Could you check a few things on this model? Use its own coordinates, in mm. Face numbers are marked on the shaded views. A direction names the side the tool comes from. Round coordinates to 2 decimals unless told otherwise and drop trailing zeros. Loops run counter-clockwise (first coordinate to the right, second up) from the corner with the lowest first, then second, coordinate; pieces in that order, holes last.
from build123d import *

# Parameters (mm, degrees)
BOSS_EXTRUDE1_DEPTH = 20
SKETCH5_W           = 39
SKETCH5_H           = 32
CUT_EXTRUDE1_DEPTH  = 98.75607398
SKETCH6_W           = 59
SKETCH6_H           = 54.995658629
CUT_EXTRUDE2_DEPTH  = 15
SKETCH7_W           = 115
SKETCH7_H           = 80
CUT_EXTRUDE3_DEPTH  = 15
SKETCH8_OUTSIDE_W   = 145.484
SKETCH8_OUTSIDE_H   = 60.484
CUT_EXTRUDE4_DEPTH  = 170.576678821


with BuildPart() as part:
    # Sketch1 → Boss-Extrude1 (new body)
    with BuildSketch(Plane(origin=(0, 0, 0), x_dir=(1, 0, 0), z_dir=(0, 1, 0))):
        with BuildLine():
            Line((40, -52.5), (-40, -52.5))
            ThreePointArc((-40, -52.5), (-68.284271247, -40.784271247), (-80, -12.5))
            Line((-80, -12.5), (-80, 12.5))
            ThreePointArc((-80, 12.5), (-68.284271247, 40.784271247), (-40, 52.5))
            Line((-40, 52.5), (40, 52.5))
            ThreePointArc((40, 52.5), (68.284271247, 40.784271247), (80, 12.5))
            Line((80, 12.5), (80, -12.5))
            ThreePointArc((80, -12.5), (68.284271247, -40.784271247), (40, -52.5))
        make_face()
    extrude(amount=BOSS_EXTRUDE1_DEPTH)

    # Sketch5 → Cut-Extrude1 (cut, through all)
    with BuildSketch(Plane(origin=(0, 20, 0), x_dir=(1, 0, 0), z_dir=(0, 1, 0))):
        with Locations((-0.079334532, -24.5)):
            Rectangle(SKETCH5_W, SKETCH5_H)
    extrude(amount=-CUT_EXTRUDE1_DEPTH, mode=Mode.SUBTRACT)

    # Sketch6 → Cut-Extrude2 (cut)
    with BuildSketch(Plane.XZ):
        with Locations((-0.079334532, 15.997829315)):
            Rectangle(SKETCH6_W, SKETCH6_H)
    extrude(amount=-CUT_EXTRUDE2_DEPTH, mode=Mode.SUBTRACT)

    # Sketch7 → Cut-Extrude3 (cut)
    with BuildSketch(Plane.XZ):
        Rectangle(SKETCH7_W, SKETCH7_H)
    extrude(amount=-CUT_EXTRUDE3_DEPTH, mode=Mode.SUBTRACT)

    # Sketch8 outside → Cut-Extrude4 (cut, through all)
    with BuildSketch(Plane(origin=(80, 0, 0), x_dir=(0, 0, -1), z_dir=(1, 0, 0))):
        with Locations((0, 10)):
            Rectangle(SKETCH8_OUTSIDE_W, SKETCH8_OUTSIDE_H)
        Polygon((0, 20), (52.5, 7.5), (52.5, 0), (-27.5, 0), (-52.5, 0), (-52.5, 20), (-27.5, 20), align=None, mode=Mode.SUBTRACT)
    extrude(amount=-CUT_EXTRUDE4_DEPTH, mode=Mode.SUBTRACT)


solid = part.part
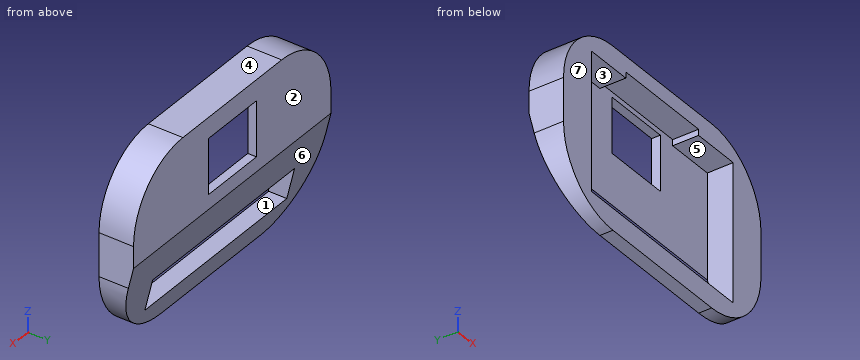
Item 1: Will these pins go through, and if not, where does the flat tip stop? pin 1 (4.5 mm diameter, centred on x = -44, y = 6.5, fed in from -Z); pin 2 (4 mm diameter, centred on y = 16.5, z = 26, fed in from +X); pin 3 (12 mm diameter, centred on y = 16, z = 38.5, fed in from -X).
Results list:
pin 1: stops at z = -52.46
pin 2: stops at x = 78.31
pin 3: stops at x = -74.64
Item 2: If we section it at B-B, the plane x = -37.5: Please give me the cut outline in (y, z).
Results list:
outline: (0, -52.5) - (7.5, -52.5) - (10.48, -40) - (0, -40) - close; (0, 40) - (15, 40) - (15, -21) - (20, 0) - (20, 52.5) - (0, 52.5) - close
Item 3: For the marked faces 1, 2 and 3, which set-ups out of +Z, -Z, +X, -X, +Y, -Y let a thin tool reach every point of the face, with its end or its side?
Results list:
face 1: +Y, -Y
face 2: +Z, -Z, +X, -X, +Y
face 3: -Y
Item 4: If we section it at A-A, the plane x = 4: Please give me the cut outline in (y, z), then the cut area to 3 significant figures.
Results list:
outline: (0, -52.5) - (7.5, -52.5) - (10.48, -40) - (0, -40) - close; (0, 43.5) - (15, 43.5) - (15, 40.5) - (20, 40.5) - (20, 52.5) - (0, 52.5) - close; (15, -21) - (20, 0) - (20, 8.5) - (15, 8.5) - close
area: 402 mm2
Item 5: If we section it at D-D, the plane z = -35: Please give me the cut outline in (x, y).
Results list:
outline: (-73.07, 0) - (-57.5, 0) - (-57.5, 11.67) - (-73.07, 11.67) - close; (57.5, 0) - (73.07, 0) - (73.07, 11.67) - (57.5, 11.67) - close
Item 6: If we section it at C-C, the plane y = 2.5: Please give me the cut outline in (x, z), then the cut area to 3 significant figures.
Results list:
outline: (-80, -12.5) arc R40 ccw to (-40, -52.5) - (40, -52.5) arc R40 ccw to (80, -12.5) - (80, 12.5) arc R40 ccw to (40, 52.5) - (-40, 52.5) arc R40 ccw to (-80, 12.5) - close; hole (-57.5, -40) - (57.5, -40) - (57.5, 40) - (29.42, 40) - (29.42, 43.5) - (-29.58, 43.5) - (-29.58, 40) - (-57.5, 40) - close
area: 6,020 mm2
Item 7: If I drill on line 1 along X through (y, z) = (3.75, 6.5); line 2 along Z through (x, y) = (-25, 2.5); line 3 along X through (y, z) = (10.5, -26), over which ranges is the centre line in solid material (lowest first)?
Results list:
line 1: x = -80 to -57.5, 57.5 to 80
line 2: z = -52.5 to -40, 43.5 to 52.5
line 3: x = -77.65 to -57.5, 57.5 to 77.65
Item 8: We'd pull the mould along Z, two halves only. Please class the marked faces 4, 5, 6 and 7: released by +Z, released by -Z, zero draft, split by the parting line, or undercut.
Results list:
face 4: released by +Z
face 5: undercut
face 6: released by -Z
face 7: zero draft
